For this review, use the dimensioned drawing (mm, ordinates from the lowest corner) and the shaded views. Coordinates: 2 decimals unless noted, no trailing zeros. Order: outer loops, then holes, each group sorted by start corner. A loop starts at its lowest first (then second) coordinate and runs counter-clockwise, first axis right, second up. Notation, with made-up numbers: M 86.5,8.5 L 117.5,8.5 A16 ccw 117.5,30.5 Z; hole C 71,29 d4. An arc over 180 degrees is marked long. Answer as CSV lines item,"result". Start each with the question number.
Q1. Consider section D-D on y = 13. Write out the cut boundary in (x, z) (1 decimal), and give its area (3 significant figures).
Q2. The part is to be moulded in two halves that separate along X. For the marked faces 1, 2, 3 and 4, say which applies: +X half, -X half, draft (parallel to the pull), parting line (faces both ways), or undercut.
Q3. Wall thickness on L1, parallel to X at y = 10.75, z = 1.7 (1 decimal); L2, parallel to X at y = 4, z = 0.7 (1 decimal): over which ranges is each line inside the solid? List them lowest first. Write a range as [from, to].
Q4. Consider section A-A on x = 7. Write out the cut boundary in (y, z) (1 decimal), and give its area (3 significant figures).
Q5. For P1, Ø3, axis at x = 7, y = 8.5, coming from the -Z side; P2, Ø1.5, axis at y = 10.5, z = 1, coming from the -X side, all flat-tipped, find the tip position at first contact; note any pin that passes through.
Q6. Consider section C-C on z = 0.65. Write out the cut boundary in (x, y) (1 decimal).
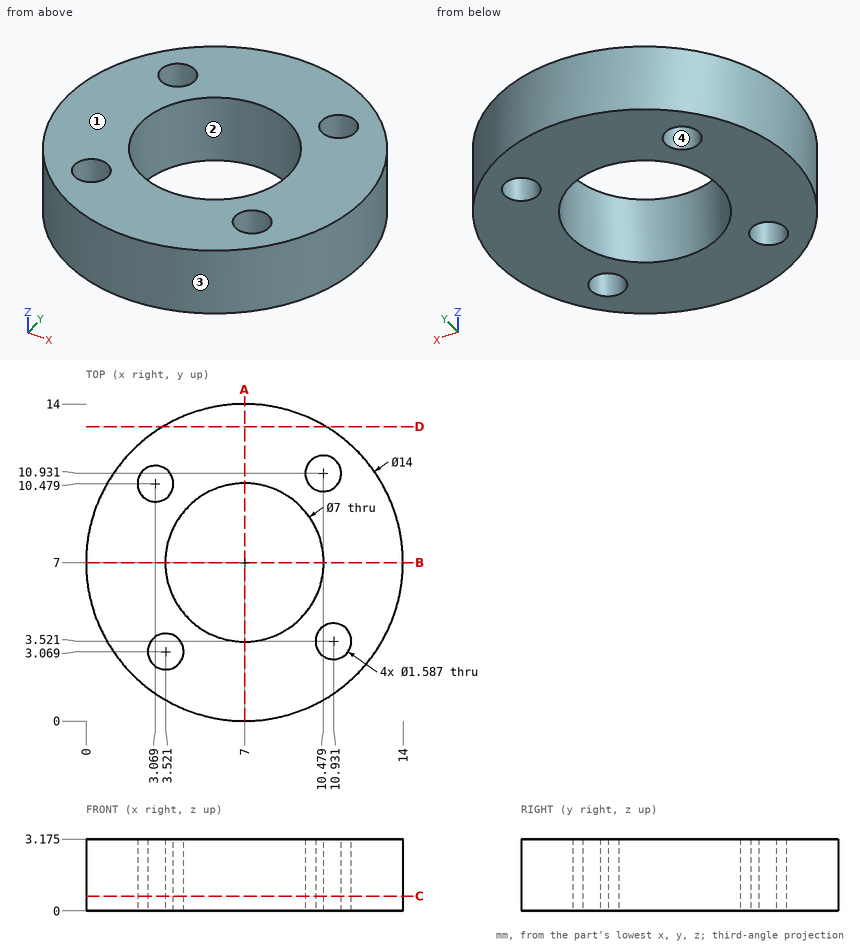
Evaluation:
1,outline,"M 3.4,0 L 10.6,0 L 10.6,3.2 L 3.4,3.2 Z"
1,area,"22.9 mm²"
2,face 1,"draft"
2,face 2,"undercut"
2,face 3,"parting line"
2,face 4,"undercut"
3,L1,"x = [1.1, 2.3], [3.8, 9.7], [11.3, 12.9]"
3,L2,"x = [0.7, 5.2], [8.8, 10.3], [11.6, 13.3]"
4,outline,"M 0,0 L 3.5,0 L 3.5,3.2 L 0,3.2 Z; M 10.5,0 L 14,0 L 14,3.2 L 10.5,3.2 Z"
4,area,"22.2 mm²"
5,P1,"passes through"
5,P2,"stops at x = 0.56"
6,outline,"C 7,7 d14; hole C 3.1,10.5 d1.6; hole C 3.5,3.1 d1.6; hole C 7,7 d7; hole C 10.5,10.9 d1.6; hole C 10.9,3.5 d1.6"
